Design review of the part shown in the three views and the two pictorial views. Dimensions are in mm from the part's minimum x, y and z. A direction names the side the tool comes from. Coordinates: 2 decimals unless noted, no trailing zeros. Write each loop counter-clockwise with the first axis right and the second up, starting at its lowest first coordinate (ties: lowest second). Pieces come first, ordered by that corner, then holes.
Q1. For the marked faces 4 and 5, list the 3-axis set-ups (+Z, -Z, +X, -X, +Y, -Y) from which the entire face can be reached by the end or side of a thin tool; tool diameter is ignored.
Q2. Take a section at B-B, the plane x = 17.5. Write out the cut boundary in (y, z) (1 decimal).
Q3. The part is to be moulded in two halves that separate along Y. For the marked faces 1, 2 and 3, say which applies: released by +Y, released by -Y, zero draft, split by the parting line, or undercut.
Q4. Take a section at A-A, the plane y = 7.75. Write out the cut boundary in (x, z) (1 decimal).
Q5. Take a section at C-C, the plane z = 4. Write out the cut boundary in (x, y) (1 decimal).
Q6. Take a section at D-D, the plane x = 5.5. Write out the cut boundary in (y, z) (1 decimal).
Q7. For L1, parallel to Y at x = 19, z = 8 (1 decimal); L2, parallel to X at y = 7.75, z = 13 (1 decimal); L3, parallel to Y at x = 6, z = 23.25 (1 decimal), list the stretches that pass through material, from the lowest coordinate up.
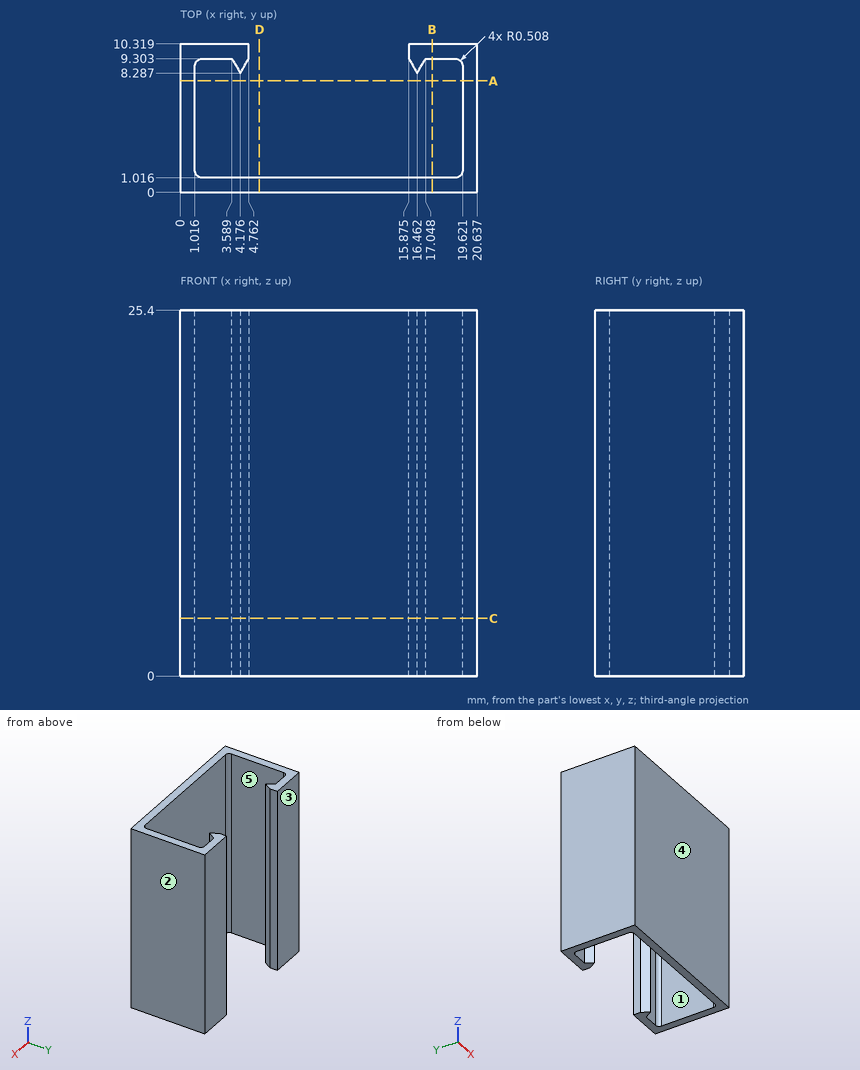
Responses:
1. face 4: +Z, -Z, +X, -X, -Y
1. face 5: +Z, -Z
2. outline: (0, 0) - (1, 0) - (1, 25.4) - (0, 25.4) - close; (9.3, 0) - (10.3, 0) - (10.3, 25.4) - (9.3, 25.4) - close
3. face 1: undercut
3. face 2: zero draft
3. face 3: released by +Y
4. outline: (0, 0) - (1, 0) - (1, 25.4) - (0, 25.4) - close; (19.6, 0) - (20.6, 0) - (20.6, 25.4) - (19.6, 25.4) - close
5. outline: (0, 0) - (20.6, 0) - (20.6, 10.3) - (15.9, 10.3) - (15.9, 9.3) - (16.5, 8.3) - (17, 9.3) - (19.1, 9.3) arc R0.5 cw to (19.6, 8.8) - (19.6, 1.5) arc R0.5 cw to (19.1, 1) - (1.5, 1) arc R0.5 cw to (1, 1.5) - (1, 8.8) arc R0.5 cw to (1.5, 9.3) - (3.6, 9.3) - (4.2, 8.3) - (4.8, 9.3) - (4.8, 10.3) - (0, 10.3) - close
6. outline: (0, 0) - (1, 0) - (1, 25.4) - (0, 25.4) - close
7. L1: y = 0 to 1, 9.3 to 10.3
7. L2: x = 0 to 1, 19.6 to 20.6
7. L3: y = 0 to 1
